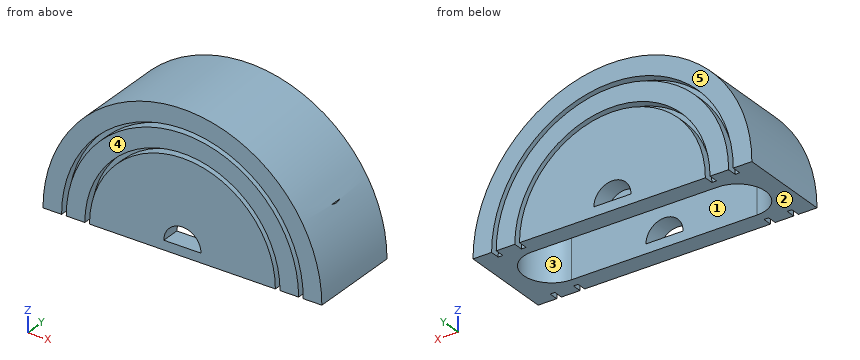
from build123d import *

# Parameters (mm, degrees)
EXTRUDE_1_DEPTH     = 5
CUT_EXTRUDE_2_DEPTH = 1
CUT_EXTRUDE_3_DEPTH = 1
CUT_EXTRUDE_4_DEPTH = 7.5
CUT_EXTRUDE_5_DEPTH = 2


with BuildPart() as part:
    # 草图1 → 凸台-拉伸1 (new, symmetric)
    with BuildSketch(Plane(origin=(0, 0, 0), x_dir=(1, 0, 0), z_dir=(0, 1, 0))):
        with BuildLine():
            Line((0, 0), (30, 0))
            ThreePointArc((30, 0), (15, -15), (0, 0))
        make_face()
    extrude(amount=EXTRUDE_1_DEPTH, both=True)

    # 草图2 → 切除-拉伸2 (cut)
    with BuildSketch(Plane.XZ.offset(5)):
        with BuildLine():
            Line((2, 0), (2.5, 0))
            ThreePointArc((2.5, 0), (15, 12.5), (27.5, 0))
            Line((27.5, 0), (28, 0))
            ThreePointArc((28, 0), (15, 13), (2, 0))
        make_face()
    cut_extrude_2 = extrude(amount=-CUT_EXTRUDE_2_DEPTH, mode=Mode.SUBTRACT)

    # 草图3 → 切除-拉伸3 (cut)
    with BuildSketch(Plane.XZ.offset(5)):
        with BuildLine():
            Line((4.5, 0), (5, 0))
            ThreePointArc((5, 0), (15, 10), (25, 0))
            Line((25, 0), (25.5, 0))
            ThreePointArc((25.5, 0), (15, 10.5), (4.5, 0))
        make_face()
    cut_extrude_3 = extrude(amount=-CUT_EXTRUDE_3_DEPTH, mode=Mode.SUBTRACT)

    # 镜向1: 切除-拉伸2, 切除-拉伸3 across plane
    add(cut_extrude_2.mirror(Plane(origin=(0, 0, 0), x_dir=(0, 0, 1), z_dir=(0, -1, 0))), mode=Mode.SUBTRACT)
    add(cut_extrude_3.mirror(Plane(origin=(0, 0, 0), x_dir=(0, 0, 1), z_dir=(0, -1, 0))), mode=Mode.SUBTRACT)

    # 草图5 → 切除-拉伸4 (cut)
    with BuildSketch(Plane(origin=(0, 0, 0), x_dir=(-1, 0, 0), z_dir=(0, 0, -1))):
        with BuildLine():
            Line((-25.030175513, -3), (-5.030175513, -3))
            ThreePointArc((-5.030175513, -3), (-2.01419916, 0.015976353), (-5.030175513, 3.031952706))
            Line((-5.030175513, 3.031952706), (-25.030175513, 3.031952706))
            ThreePointArc((-25.030175513, 3.031952706), (-28.046151866, 0.015976353), (-25.030175513, -3))
        make_face()
    extrude(amount=-CUT_EXTRUDE_4_DEPTH, mode=Mode.SUBTRACT)

    # 草图6 → 切除-拉伸5 (cut)
    with BuildSketch(Plane.XZ.offset(5)):
        with BuildLine():
            Line((13, 1), (17, 1))
            ThreePointArc((17, 1), (15, 3), (13, 1))
        make_face()
    cut_extrude_5 = extrude(amount=-CUT_EXTRUDE_5_DEPTH, mode=Mode.SUBTRACT)

    # 镜向2: 切除-拉伸5 across plane
    add(cut_extrude_5.mirror(Plane(origin=(0, 0, 0), x_dir=(0, 0, 1), z_dir=(0, -1, 0))), mode=Mode.SUBTRACT)


solid = part.part
For this review, take the finished solid that the model builds, in its own axes (mm). Face numbers are marked on the shaded views. A direction names the side the tool comes from. Round coordinates to 2 decimals unless told otherwise and drop trailing zeros. Write each loop counter-clockwise with the first axis right and the second up, starting at its lowest first coordinate (ties: lowest second). Pieces come first, ordered by that corner, then holes. Notation, with made-up numbers: (-18, 84.5) -> (4, 84.5) arc R16 ccw to (4, 115.5) -> close; hole circle Ø9 at (-3, 9). An arc over 180 degrees is marked (long way). Put each result on its own line as item: value.
Q1. Consider section B-B on x = 3.5. State the section outline as (y, z) points, and give its area (3 significant figures).
Determined:
outline: (-5, 0) -> (-2.58, 0) -> (-2.58, 7.5) -> (2.61, 7.5) -> (2.61, 0) -> (5, 0) -> (5, 4.9) -> (4, 4.9) -> (4, 6.06) -> (5, 6.06) -> (5, 9.63) -> (-5, 9.63) -> (-5, 6.06) -> (-4, 6.06) -> (-4, 4.9) -> (-5, 4.9) -> close
area: 55.0 mm^2
Q2. Consider section D-D on x = 11.5. State the section outline as (y, z) points, and give its area (3 significant figures).
Determined:
outline: (-5, 0) -> (-3, 0) -> (-3, 7.5) -> (3.03, 7.5) -> (3.03, 0) -> (5, 0) -> (5, 9.37) -> (4, 9.37) -> (4, 9.9) -> (5, 9.9) -> (5, 12) -> (4, 12) -> (4, 12.52) -> (5, 12.52) -> (5, 14.59) -> (-5, 14.59) -> (-5, 12.52) -> (-4, 12.52) -> (-4, 12) -> (-5, 12) -> (-5, 9.9) -> (-4, 9.9) -> (-4, 9.37) -> (-5, 9.37) -> close
area: 98.5 mm^2
Q3. The part is to be moulded in two halves that separate along Y. For the marked faces 3, 4 and 5, say which applies: released by +Y, released by -Y, zero draft, split by the parting line, or undercut.
Determined:
face 3: undercut
face 4: released by -Y
face 5: released by +Y
Q4. To check wall thickness, follow L1, parallel to Y at x = 21.5, z = 6.5; L2, parallel to X at y = -4.5, z = 3.5; L3, parallel to X at y = -4.5, z = 4.5. State the ranges of each line that lie inside material, in increasing order. Write a range as [from, to].
Determined:
L1: y = [-5, -3], [3.03, 5]
L2: x = [0.41, 2.48], [3, 5.1], [5.63, 24.37], [24.9, 27], [27.52, 29.59]
L3: x = [0.69, 2.8], [3.34, 5.51], [6.07, 23.93], [24.49, 26.66], [27.2, 29.31]
Q5. Consider section A-A on x = 15. Give the number of separate pieces and of enclosed holes in the cut face, and give its area (3 significant figures).
Determined:
separate pieces: 3
enclosed holes: 0
area: 94.8 mm^2
Q6. Machinability: for the marked faces 1 and 2, which of the approach directions +Z, -Z, +X, -X, +Y, -Y give a long, thin tool a straight path to every point of the face, cutting with its end or side? Answer none if there is none.
Determined:
face 1: -Z
face 2: -Z, +X, -X, +Y, -Y
Q7. Clearance check with flat-ended pins moving along their axes: pin 1 Ø1 at (x, y) = (14, 4) entering from +Z; pin 2 Ø4 at (x, z) = (14.5, 2.5) entering from +Y; pin 3 Ø2 at (y, z) = (-1, 10) entering from -X; pin 4 Ø1.8 at (x, y) = (14, 1) entering from -Z. State where each tip first meets the part, or that it passes through.
Determined:
pin 1: stops at z = 14.99
pin 2: stops at y = 5
pin 3: stops at x = 3
pin 4: stops at z = 7.5
Q8. Consider section C-C on y = 2.5. State the section outline as (x, z) points, and give its area (3 significant figures).
Determined:
outline: (0, 0) -> (3.32, 0) -> (3.32, 7.5) -> (26.74, 7.5) -> (26.74, 0) -> (30, 0) arc R15 ccw to start
area: 178 mm^2
